Read the model definition and answer for the solid it produces. Units are mm, in the model's axes. Round coordinates to 2 decimals unless told otherwise and drop trailing zeros. Write each loop counter-clockwise with the first axis right and the second up, starting at its lowest first coordinate (ties: lowest second). Pieces come first, ordered by that corner, then holes.
from build123d import *

# Parameters (mm, degrees)
SKETCH1_W                     = 50.8
SKETCH1_H                     = 9.525
BOSS_EXTRUDE1_DEPTH           = 118.775
TAP_DRILL_FOR_M3X0_5_TAP1_D   = 2.5
CSK_FOR_M4_SFHCS1_D           = 4.5
CSK_FOR_M4_SFHCS1_CSINK_D     = 8.96
CSK_FOR_M4_SFHCS1_CSINK_ANGLE = 90


with BuildPart() as part:
    # Sketch1 → Boss-Extrude1 (new, symmetric)
    with BuildSketch(Plane.XY):
        Rectangle(SKETCH1_W, SKETCH1_H)
    extrude(amount=BOSS_EXTRUDE1_DEPTH, both=True)

    # Tap Drill for M3x0.5 Tap1 (through all)
    with Locations(Plane(origin=(0, 4.7625, 0), x_dir=(1, 0, 0), z_dir=(0, 1, 0))):
        with Locations((-15, 98.775), (15, 98.775), (-15, 83.775), (15, 83.775), (15, 13.775), (-15, 13.775), (15, -1.225), (-15, -1.225)):
            Hole(TAP_DRILL_FOR_M3X0_5_TAP1_D / 2)

    # CSK for M4 SFHCS1 (through all)
    with Locations(Plane(origin=(0, 4.7625, 0), x_dir=(1, 0, 0), z_dir=(0, 1, 0))):
        with Locations((-20, -104.25), (20, -104.25)):
            CounterSinkHole(CSK_FOR_M4_SFHCS1_D / 2, CSK_FOR_M4_SFHCS1_CSINK_D / 2, counter_sink_angle=CSK_FOR_M4_SFHCS1_CSINK_ANGLE)


solid = part.part
Q1. Section A-A (x = 20) is taken. Determine the outline of the cut face in (y, z) (1 decimal).
Verdict:
outline: (-4.8, -118.8) - (4.8, -118.8) - (4.8, 99.8) - (2.5, 102) - (-4.8, 102) - close; (-4.8, 106.5) - (2.5, 106.5) - (4.8, 108.7) - (4.8, 118.8) - (-4.8, 118.8) - close
Q2. Straight lines are drawn through the part: probe 1 along X at (y, z) = (1, 104.25); probe 2 along Z at (x, y) = (-15, 1) (3 decimals); probe 3 along Z at (x, y) = (-20, 0.75) (3 decimals). For each, find the intervals that lie inside material, in ascending order.
Verdict:
probe 1: x = -25.4 to -22.25, -17.75 to 17.75, 22.25 to 25.4
probe 2: z = -118.775 to -100.025, -97.525 to -85.025, -82.525 to -15.025, -12.525 to -0.025, 2.475 to 118.775
probe 3: z = -118.775 to 102, 106.5 to 118.775
Q3. Flat-ended cylindrical pins translate along their axes: pin 1 Ø6 at (x, z) = (-20, 104.25) entering from -Y; pin 2 Ø5 at (x, z) = (20, 104.25) entering from +Y. Find the tip coordinate at first contact, or state that the pin passes through.
Verdict:
pin 1: stops at y = -4.76
pin 2: stops at y = 2.78
